Geometry check sheet. Reference: drawing and pictorial views, mm from the part's lowest x, y, z. A direction names the side the tool comes from. Coordinates: 2 decimals unless noted, no trailing zeros. Write each loop counter-clockwise with the first axis right and the second up, starting at its lowest first coordinate (ties: lowest second). Pieces come first, ordered by that corner, then holes.
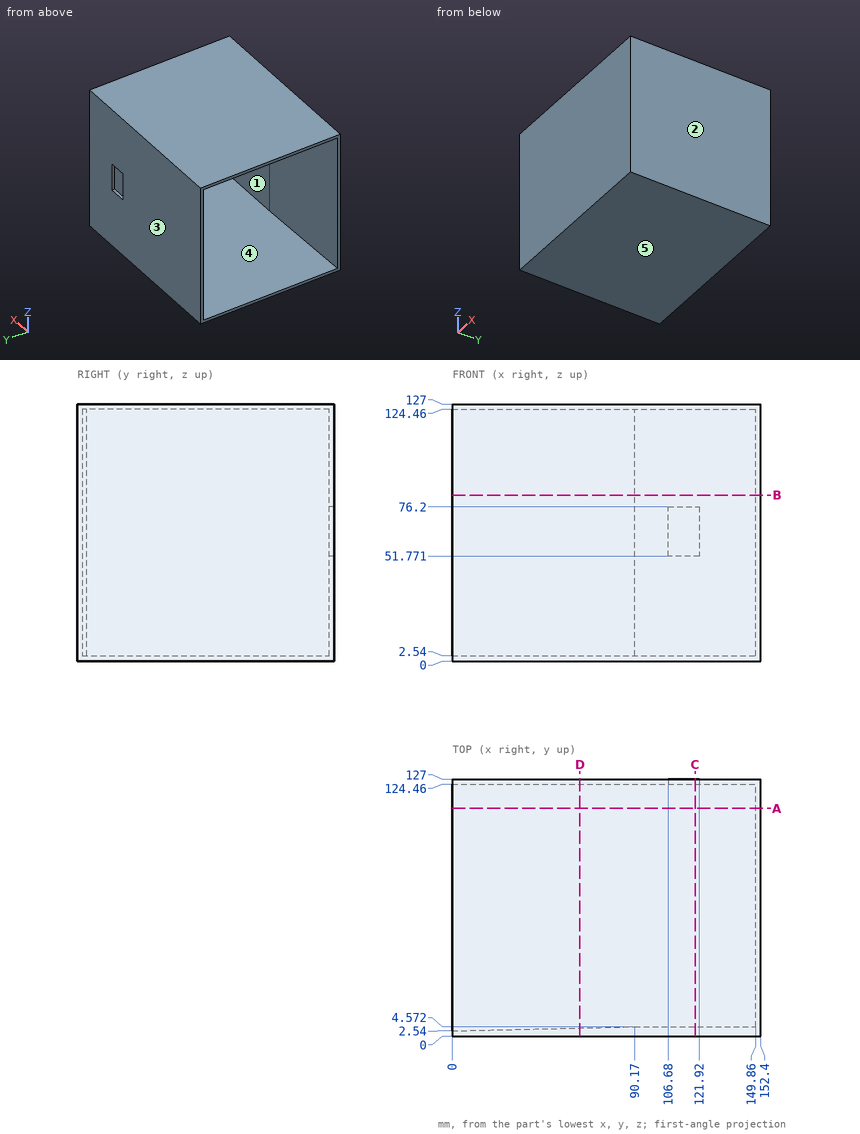
1. Sectioned sample at D-D, the plane x = 63. Record the boundary of the cut face in (y, z).
2. Tool access check on the marked faces 4 and 5. Record the directions out of +Z, -Z, +X, -X, +Y, -Y that give a thin tool (end or side, any length) a straight path to the whole face; none if there is none.
3. Sectioned sample at B-B, the plane z = 82. Record the boundary of the cut face in (x, y).
4. Sectioned sample at C-C, the plane x = 120. Record the boundary of the cut face in (y, z), and give its area (3 significant figures).
5. Material ranges on L1, parallel to Z at x = 143, y = 12.5; L2, parallel to X at y = 55, z = 50; L3, parallel to Y at x = 136, z = 39.5, recorded low to high.
6. Gauge pin test, flat ends, axial feed: P1, Ø1.3, axis at x = 116, y = 125.5, coming from the -Z side; P2, Ø1.5, axis at y = 42, z = 90, coming from the -X side. Record the tip position at first contact, or that the pin passes through.
7. Draft check along Y on the marked faces 1, 2 and 3. Enter one of: pulls with the +Y half, pulls with the -Y half, needs draft (parallel to the pull), parting line crosses it, or undercut.
8. Sectioned sample at A-A, the plane y = 112.5. Record the boundary of the cut face in (x, z), and give its area (3 significant figures).
Outcome:
1. outline: (0, 0) - (127, 0) - (127, 127) - (0, 127) - close; hole (3.96, 2.54) - (124.46, 2.54) - (124.46, 124.46) - (3.96, 124.46) - close
2. face 4: -X
2. face 5: -Z, +X, -X, +Y, -Y
3. outline: (0, 0) - (152.4, 0) - (152.4, 127) - (0, 127) - (0, 124.46) - (149.86, 124.46) - (149.86, 4.57) - (90.17, 4.57) - (0, 2.54) - close
4. outline: (0, 0) - (127, 0) - (127, 51.77) - (124.46, 51.77) - (124.46, 2.54) - (4.57, 2.54) - (4.57, 124.46) - (124.46, 124.46) - (124.46, 76.2) - (127, 76.2) - (127, 127) - (0, 127) - close
4. area: 1,450 mm2
5. L1: z = 0 to 2.54, 124.46 to 127
5. L2: x = 149.86 to 152.4
5. L3: y = 0 to 4.57, 124.46 to 127
6. P1: stops at z = 0
6. P2: stops at x = 149.86
7. face 1: undercut
7. face 2: needs draft
7. face 3: pulls with the +Y half
8. outline: (0, 0) - (152.4, 0) - (152.4, 127) - (0, 127) - (0, 124.46) - (149.86, 124.46) - (149.86, 2.54) - (0, 2.54) - close
8. area: 1,080 mm2
